```python
from build123d import *

# Parameters (mm, degrees)
PAD_DEPTH       = 40
FILLET_R        = 1
FILLET001_R     = 3
SKETCH001_R     = 3
POCKET_DEPTH    = 40.001
POCKET001_DEPTH = 100.001
SKETCH004_R     = 3
POCKET002_DEPTH = 40.001


with BuildPart() as part:
    # Sketch → Pad (new body)
    with BuildSketch(Plane.XY):
        Polygon((-14.945557, 10.4), (-20.95, 0), (20.95, 0), (14.945557, 10.4), (50, 10.4), (50, -15), (-50, -15), (-50, 10.4), align=None)
    extrude(amount=PAD_DEPTH)

    # Fillet
    fillet_edges = [part.edges().sort_by_distance(p)[0] for p in [
        (20.95, 0, 20),
        (-20.95, 0, 20),
        (-14.945557, 10.4, 20),
        (14.945557, 10.4, 20),
    ]]
    fillet(fillet_edges, radius=FILLET_R)

    # Fillet001
    fillet001_edges = [part.edges().sort_by_distance(p)[0] for p in [
        (-50, 10.4, 20),
        (50, 10.4, 20),
        (50, -15, 20),
        (-50, -15, 20),
    ]]
    fillet(fillet001_edges, radius=FILLET001_R)

    # Sketch001 → Pocket (cut, through all)
    with BuildSketch(Plane(origin=(0, 0, 0), x_dir=(1, 0, 0), z_dir=(0, 0, -1))):
        with Locations((0, 8)):
            Circle(SKETCH001_R)
    extrude(amount=-POCKET_DEPTH, mode=Mode.SUBTRACT)

    # Sketch002 → Pocket001 (cut, through all)
    with BuildSketch(Plane(origin=(-50, 0, 0), x_dir=(0, -1, 0), z_dir=(-1, 0, 0))):
        Polygon((2.157222, 14.193818), (-4.913846, 21.264885), (2.157222, 28.335953), (9.22829, 21.264885), align=None)
    extrude(amount=-POCKET001_DEPTH, mode=Mode.SUBTRACT)

    # Sketch004 → Pocket002 (cut, through all)
    with BuildSketch(Plane.XY.offset(40)):
        with Locations((-36.544449, -2.244335)):
            Circle(SKETCH004_R)
    extrude(amount=-POCKET002_DEPTH, mode=Mode.SUBTRACT)


solid = part.part
```
Model file for the job. Use its own axes, mm. A direction names the side the tool comes from. Give positions to 0.01 mm unless a question says otherwise; leave off trailing zeros. Loops run counter-clockwise (first coordinate to the right, second up) from the corner with the lowest first, then second, coordinate; pieces in that order, holes last. Notation, with made-up numbers: (52, 59) -> (62, 59) arc R9 cw to (62, 76) -> close; hole circle Ø3 at (36.5, -9). An arc over 180 degrees is marked (long way). Use CSV: the item, a comma, the result in double quotes. Start each with the question number.
1) Slice it at C-C on z = 3. Give the cut face in (x, y), plus the area to 3 significant figures.
2) Slice it at D-D on x = -38.5. Give the cut face in (y, z), plus the area to 3 significant figures.
3) Wall check: line 1 (Y direction, x = 0, z = 28.5); line 2 (X direction, y = -2.5, z = 34); line 3 (X direction, y = -8, z = 17). Give the ranges that are in metal, low to high.
4) Slice it at B-B on y = -4. Give the cut face in (x, z), plus the area to 3 significant figures.
5) Flat gauge pins, fed straight in: pin 1 Ø11 at (x, z) = (0, 34) entering from +Y; pin 2 Ø12 at (x, y) = (-14.5, -9) entering from -Z; pin 3 Ø5.5 at (x, y) = (-36.54, -2.24) entering from -Z. Where does each tip first touch, or does it go through?
6) Slice it at A-A on x = 0. Give the cut face in (y, z), plus the area to 3 significant figures.
7) Tool access for faces 5 (the flat face through (-17.92, 5.25, 19.72)), 6 (the flat face through (-0.7, -0.24, 16.11)), 7 (the cylindrical face through (-49.1, 9.54, 20.28)): list every direction of +Z, -Z, +X, -X, +Y, -Y with a clear straight run to the whole face (end or side of a thin tool).
8) Mould opens along Z. For faces 1 (the cylindrical face through (-49.14, -14.1, 20.28)), 2 (the flat face through (-0.7, -4.858, 25.636)), 3 (the flat face through (-0.7, -4.171, 16.208)), 4 (the flat face through (1, -2, 40)) say: released by +Z, released by -Z, zero draft, split by the parting line, or undercut.
Computed values:
1,outline,"(-50, -12) arc R3 ccw to (-47, -15) -> (47, -15) arc R3 ccw to (50, -12) -> (50, 7.4) arc R3 ccw to (47, 10.4) -> (16.68, 10.4) arc R1 ccw to (15.81, 8.9) -> (20.08, 1.5) arc R1 cw to (19.22, 0) -> (-19.22, 0) arc R1 cw to (-20.08, 1.5) -> (-15.81, 8.9) arc R1 ccw to (-16.68, 10.4) -> (-47, 10.4) arc R3 ccw to (-50, 7.4) -> close; hole circle Ø6 at (-36.54, -2.24); hole circle Ø6 at (0, -8)"
1,area,"2,100 mm^2"
2,outline,"(-15, 0) -> (-4.52, 0) -> (-4.52, 16.56) -> (-9.23, 21.26) -> (-4.52, 25.97) -> (-4.52, 40) -> (-15, 40) -> close; (0.03, 0) -> (10.4, 0) -> (10.4, 40) -> (0.03, 40) -> (0.03, 26.15) -> (4.91, 21.26) -> (0.03, 16.38) -> close"
2,area,"788 mm^2"
3,line 1,"y = -15 to -11, -5 to 0"
3,line 2,"x = -50 to -39.53, -33.56 to 50"
3,line 3,"x = -50 to -3, 3 to 50"
4,outline,"(-50, 0) -> (-38.98, 0) -> (-38.98, 16.04) -> (-50, 16.04) -> close; (-50, 26.49) -> (-38.98, 26.49) -> (-38.98, 40) -> (-50, 40) -> close; (-34.11, 0) -> (50, 0) -> (50, 16.04) -> (-34.11, 16.04) -> close; (-34.11, 26.49) -> (50, 26.49) -> (50, 40) -> (-34.11, 40) -> close"
4,area,"2,810 mm^2"
5,pin 1,"stops at y = 0"
5,pin 2,"stops at z = 0"
5,pin 3,"passes through"
6,outline,"(-15, 0) -> (-11, 0) -> (-11, 40) -> (-15, 40) -> close; (-5, 0) -> (0, 0) -> (0, 16.35) -> (-2.16, 14.19) -> (-5, 17.04) -> close; (-5, 25.49) -> (-2.16, 28.34) -> (0, 26.18) -> (0, 40) -> (-5, 40) -> close"
6,area,"302 mm^2"
7,face 5,"+Z, -Z"
7,face 6,"+X, -X"
7,face 7,"+Z, -Z, -X, +Y"
8,face 1,"zero draft"
8,face 2,"undercut"
8,face 3,"undercut"
8,face 4,"released by +Z"
